from build123d import *

# Parameters (mm, degrees)
F0_W     = 50
F0_H     = 30
F1_DEPTH = 5
F2_R     = 1.8
F3_DEPTH = 5.001
F4_R     = 1.8
F4_R_2   = 2.25
F5_DEPTH = 5.001
F6_R     = 1.8
F7_DEPTH = 5.001


with BuildPart() as f1:
    # F0 (on Front) → F1 (new body)
    with BuildSketch(Plane.XZ):
        Rectangle(F0_W, F0_H)
    extrude(amount=F1_DEPTH)

    # F2 (on face) → F3 (cut, through all)
    with BuildSketch(Plane(origin=(0, 0, 0), x_dir=(-1, 0, 0), z_dir=(0, 1, 0))):
        with Locations((0, -11.5)):
            Circle(F2_R)
    extrude(amount=-F3_DEPTH, mode=Mode.SUBTRACT)

    # F4 (on face) → F5 (cut, through all)
    with BuildSketch(Plane(origin=(0, 0, 0), x_dir=(-1, 0, 0), z_dir=(0, 1, 0))):
        with Locations((8.048, -2)):
            Circle(F4_R)
        with Locations((0, -2)):
            Circle(F4_R_2)
        with Locations((-8.048, -2)):
            Circle(F4_R)
    extrude(amount=-F5_DEPTH, mode=Mode.SUBTRACT)

    # F6 (on face) → F7 (cut, through all)
    with BuildSketch(Plane(origin=(0, 0, 0), x_dir=(-1, 0, 0), z_dir=(0, 1, 0))):
        with Locations((-21, 11.5)):
            Circle(F6_R)
        with Locations((21, 11.5)):
            Circle(F6_R)
    extrude(amount=-F7_DEPTH, mode=Mode.SUBTRACT)


solid = f1.part
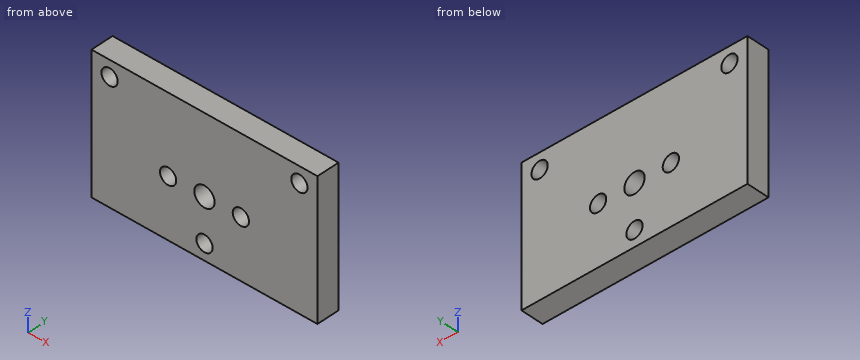
The model under review builds one solid part; all positions refer to its coordinate system, in mm. Round coordinates to 2 decimals unless told otherwise and drop trailing zeros. Loops run counter-clockwise (first coordinate to the right, second up) from the corner with the lowest first, then second, coordinate; pieces in that order, holes last. Notation, with made-up numbers: (0, -10.75) -> (49, -10.75) arc R13 ccw to (49, -2.75) -> close; hole circle Ø3 at (6.5, 54). An arc over 180 degrees is marked (long way). Write item = value, one per line. Start each with the question number.
Item 1: To check wall thickness, follow L1, parallel to Z at x = 0, y = -1.25; L2, parallel to X at y = -4.4, z = 12.75; L3, parallel to X at y = -1.2, z = 10.75. State the ranges of each line that lie inside material, in increasing order.
Item 2: Insertion check: pin 1 (2 mm diameter, centred on x = 8.048, z = -2, fed in from -Y). The pin has a flat end and moves straight along its axis. Give the tip position at first contact, or say it passes through.
Item 3: Take a section at D-D on x = 0. Give the boundary of the cut face in (y, z), plus the area to 4 significant figures.
Item 4: Take a section at A-A on z = -2. Give the boundary of the cut face in (x, y).
Item 5: Take a section at B-B on x = -21. Give the boundary of the cut face in (y, z).
Item 6: Take a section at C-C on z = -11.5. Give the boundary of the cut face in (x, y), plus the area to 3 significant figures.
Result:
q1.L1 = -15 to -13.3, -9.7 to -4.25, 0.25 to 15
q1.L2 = -25 to -22.3, -19.7 to 19.7, 22.3 to 25
q1.L3 = -25 to -22.64, -19.36 to 19.36, 22.64 to 25
q2.pin_1 = through
q3.outline = (-5, -15) -> (0, -15) -> (0, -13.3) -> (-5, -13.3) -> close; (-5, -9.7) -> (0, -9.7) -> (0, -4.25) -> (-5, -4.25) -> close; (-5, 0.25) -> (0, 0.25) -> (0, 15) -> (-5, 15) -> close
q3.area = 109.5 mm²
q4.outline = (-25, -5) -> (-9.85, -5) -> (-9.85, 0) -> (-25, 0) -> close; (-6.25, -5) -> (-2.25, -5) -> (-2.25, 0) -> (-6.25, 0) -> close; (2.25, -5) -> (6.25, -5) -> (6.25, 0) -> (2.25, 0) -> close; (9.85, -5) -> (25, -5) -> (25, 0) -> (9.85, 0) -> close
q5.outline = (-5, -15) -> (0, -15) -> (0, 9.7) -> (-5, 9.7) -> close; (-5, 13.3) -> (0, 13.3) -> (0, 15) -> (-5, 15) -> close
q6.outline = (-25, -5) -> (-1.8, -5) -> (-1.8, 0) -> (-25, 0) -> close; (1.8, -5) -> (25, -5) -> (25, 0) -> (1.8, 0) -> close
q6.area = 232 mm²
